Geometry: final body of the model. Coordinates: model frame, mm. Give positions to 0.01 mm unless a question says otherwise; leave off trailing zeros.
from build123d import *

# Parameters (mm, degrees)
BOSS_EXTRUDE1_DEPTH     = 3.175
SKETCH2_R               = 6.35
CUT_EXTRUDE1_DEPTH      = 4.1750001
CUT_EXTRUDE2_DEPTH      = 20.741500936
CUT_EXTRUDE2_DEPTH_BACK = 20.741500936


with BuildPart() as part:
    # Sketch1 → Boss-Extrude1 (new body)
    with BuildSketch(Plane.XY):
        with BuildLine():
            add(Edge.make_bspline(
                [(328.93, 0.4144518), (328.807900642, 0.516772717), (328.019000541, 0.420161926), (326.614170865, 0.815622818), (324.037900124, 1.060053788), (320.567272172, 1.584632638), (316.096583479, 2.170027594), (310.705215164, 2.891499965), (304.407193949, 3.70705594), (297.248126622, 4.61507178), (289.269853683, 5.599640546), (280.522284399, 6.647437516), (271.05918713, 7.745466949), (260.938835986, 8.878779448), (250.223661724, 10.033538187), (238.979802735, 11.195400912), (227.276553794, 12.349370833), (215.186101231, 13.479249677), (202.78290329, 14.570204468), (190.143565404, 15.603996393), (177.345750776, 16.563769435), (164.468478458, 17.43170464), (151.591090461, 18.189654233), (138.792862913, 18.818469572), (126.15283726, 19.301382712), (113.748578816, 19.622639213), (101.656743367, 19.766547691), (89.951630239, 19.721687508), (78.705404506, 19.479393557), (67.987291822, 19.033523951), (57.863264224, 18.382912366), (48.395544354, 17.529516447), (39.642067919, 16.480001255), (31.656190162, 15.24329661), (24.486303571, 13.832318834), (18.174431838, 12.263022231), (12.756441756, 10.550709399), (8.259860269, 8.711328155), (4.699027102, 6.757322776), (2.079421527, 4.684836659), (0.401585469, 2.443731656), (-0.187153107, 0), (0.401585469, -2.443731656), (2.079421527, -4.684836659), (4.699027102, -6.757322776), (8.259860269, -8.711328155), (12.756441756, -10.550709399), (18.174431838, -12.263022231), (24.486303571, -13.832318834), (31.656190162, -15.24329661), (39.642067919, -16.480001255), (48.395544354, -17.529516447), (57.863264224, -18.382912366), (67.987291822, -19.033523951), (78.705404506, -19.479393557), (89.951630239, -19.721687508), (101.656743367, -19.766547691), (113.748578816, -19.622639213), (126.15283726, -19.301382712), (138.792862913, -18.818469572), (151.591090461, -18.189654233), (164.468478458, -17.43170464), (177.345750776, -16.563769435), (190.143565404, -15.603996393), (202.78290329, -14.570204468), (215.186101231, -13.479249677), (227.276553794, -12.349370833), (238.979802735, -11.195400912), (250.223661724, -10.033538187), (260.938835986, -8.878779448), (271.05918713, -7.745466949), (280.522284399, -6.647437516), (289.269853683, -5.599640546), (297.248126622, -4.61507178), (304.407193949, -3.70705594), (310.705215164, -2.891499965), (316.096583479, -2.170027594), (320.567272172, -1.584632638), (324.037900124, -1.060053788), (326.614170865, -0.815622818), (328.019000541, -0.420161926), (329.127736254, -0.555940631), (329.127736254, 0.24874614), (328.93, 0.4144518)],
                knots=[0, 0, 0, 0, 0.000762215, 0.003044706, 0.006832246, 0.012101176, 0.018817536, 0.026939455, 0.036414848, 0.047184629, 0.059180413, 0.072327874, 0.086544061, 0.10174058, 0.117823336, 0.134691452, 0.152240154, 0.17036129, 0.188941008, 0.207865435, 0.227016078, 0.246275696, 0.265524943, 0.284644966, 0.303520118, 0.322034575, 0.340078353, 0.357542593, 0.374325482, 0.390329891, 0.40546389, 0.419643801, 0.432793371, 0.444843817, 0.455737921, 0.465428653, 0.47388632, 0.481101634, 0.487101684, 0.491975368, 0.495930678, 0.499382808, 0.502834938, 0.506790248, 0.511663932, 0.517663982, 0.524879296, 0.533336963, 0.543027695, 0.553921799, 0.565972245, 0.579121815, 0.593301726, 0.608435725, 0.624440134, 0.641223023, 0.658687263, 0.676731041, 0.695245498, 0.71412065, 0.733240673, 0.75248992, 0.771749538, 0.790900181, 0.809824608, 0.828404326, 0.846525462, 0.864074164, 0.88094228, 0.897025036, 0.912221555, 0.926437743, 0.939585203, 0.951580988, 0.962350768, 0.971826161, 0.979948081, 0.98666444, 0.991933371, 0.99572091, 0.998003402, 0.998765616, 1, 1, 1, 1], degree=3))
        make_face()
    extrude(amount=BOSS_EXTRUDE1_DEPTH)

    # Sketch2 → Cut-Extrude1 (cut, through all)
    with BuildSketch(Plane.XY.offset(3.175)):
        with Locations((88.9, 0)):
            Circle(SKETCH2_R)
        with Locations((165.1, 0)):
            Circle(SKETCH2_R)
    extrude(amount=-CUT_EXTRUDE1_DEPTH, mode=Mode.SUBTRACT)

    # Sketch3 → Cut-Extrude2 (cut, two sides)
    with BuildSketch(Plane(origin=(0, 0, 0), x_dir=(1, 0, 0), z_dir=(0, 1, 0))) as cut_extrude2_sk:
        Polygon((255.992242673, 0), (255.545593987, -3.175), (329.07830219, -3.175), (329.07830219, 0), align=None)
    extrude(amount=CUT_EXTRUDE2_DEPTH, mode=Mode.SUBTRACT)
    extrude(cut_extrude2_sk.sketch, amount=-CUT_EXTRUDE2_DEPTH_BACK, mode=Mode.SUBTRACT)

    # Sketch4 → Cut-Loft1 section 0
    with BuildSketch(Plane.XY.offset(3.175)):
        with BuildLine():
            Line((82.55, -19.515708197), (82.55, -16.251023077))
            Line((82.55, -16.251023077), (79.375, -16.251023077))
            add(Edge.make_bspline(
                [(79.375, 16.251023077), (72.770318552, 16.048049675), (66.176202719, 15.728304371), (56.30738853, 15.001567412), (53.021532705, 14.717888762), (46.459157571, 14.04734399), (43.182596705, 13.660937457), (38.276882967, 12.980450934), (36.643177419, 12.736779299), (33.379494145, 12.209172355), (31.748117674, 11.925180268), (28.498717967, 11.31067673), (26.880571377, 10.97988905), (23.660292552, 10.260780921), (22.058116365, 9.87261787), (18.875212279, 9.019251619), (17.293996052, 8.555526619), (14.162834442, 7.517257926), (12.611952901, 6.946125273), (10.325000489, 5.950076454), (9.567811499, 5.594025093), (8.461932827, 5.017489815), (8.097932617, 4.81777412), (7.381669561, 4.39922172), (7.029407018, 4.180395983), (6.339282138, 3.719594292), (6.001169966, 3.47795005), (5.346762375, 2.959692647), (5.02857237, 2.681117584), (4.439349211, 2.084395549), (4.164695388, 1.768387828), (3.820228536, 1.236176286), (3.718740433, 1.050561172), (3.59999989, 0.759299745), (3.565442077, 0.659141625), (3.509216677, 0.455376556), (3.487522742, 0.351764773), (3.459675736, 0.143592536), (3.453573255, 0.038940089), (3.461444597, -0.171798071), (3.474973766, -0.278422694), (3.536160139, -0.588423887), (3.603651886, -0.78636311), (3.780189655, -1.168677669), (3.889538593, -1.351988295), (4.129382817, -1.699026003), (4.261329389, -1.864987348), (4.67775825, -2.342961513), (4.979594961, -2.63427888), (5.614334641, -3.181856059), (5.947755344, -3.437548737), (6.980186178, -4.167859174), (7.695486627, -4.59881642), (9.156342741, -5.391257516), (9.902423269, -5.75319572), (11.414841066, -6.432708068), (12.181579116, -6.749404985), (13.73156777, -7.346635451), (14.514836956, -7.627179806), (16.093189665, -8.161972373), (16.88860874, -8.415184993), (18.482918694, -8.896317804), (19.282763312, -9.124717403), (21.688920309, -9.779957105), (23.302005405, -10.176164111), (26.541461257, -10.908476052), (28.167798474, -11.244732377), (33.062961618, -12.180447863), (36.350545365, -12.709560737), (42.938422768, -13.630876096), (46.23811967, -14.02274496), (52.84624923, -14.702163706), (56.154743063, -14.989298509), (66.090451195, -15.724271447), (72.727906329, -16.046777883), (79.375, -16.251023077)],
                knots=[0, 0, 0, 0, 0.125, 0.125, 0.1875, 0.1875, 0.25, 0.25, 0.28125, 0.28125, 0.3125, 0.3125, 0.34375, 0.34375, 0.375, 0.375, 0.40625, 0.40625, 0.4375, 0.4375, 0.453125, 0.453125, 0.4609375, 0.4609375, 0.46875, 0.46875, 0.4765625, 0.4765625, 0.484375, 0.484375, 0.4921875, 0.4921875, 0.49609375, 0.49609375, 0.498046875, 0.498046875, 0.5, 0.5, 0.501953125, 0.501953125, 0.50390625, 0.50390625, 0.5078125, 0.5078125, 0.51171875, 0.51171875, 0.515625, 0.515625, 0.5234375, 0.5234375, 0.53125, 0.53125, 0.546875, 0.546875, 0.5625, 0.5625, 0.578125, 0.578125, 0.59375, 0.59375, 0.609375, 0.609375, 0.625, 0.625, 0.65625, 0.65625, 0.6875, 0.6875, 0.75, 0.75, 0.8125, 0.8125, 0.875, 0.875, 1, 1, 1, 1], degree=3))
            Line((79.375, 16.251023077), (82.55, 16.251023077))
            Line((82.55, 16.251023077), (82.55, 19.515708197))
            Line((82.55, 19.515708197), (82.55, 26.856724286))
            Line((82.55, 26.856724286), (0.541465363, 30.021162049))
            Line((0.541465363, 30.021162049), (-2.146488993, -32.850745924))
            Line((-2.146488993, -32.850745924), (82.55, -25.525605715))
            Line((82.55, -25.525605715), (82.55, -19.515708197))
        make_face()
    # Sketch5 → Cut-Loft1 section 1
    with BuildSketch(Plane(origin=(0, 0, 0), x_dir=(-1, 0, 0), z_dir=(0, 0, -1))):
        with BuildLine():
            Line((-82.55, 16.286875084), (-82.55, 19.550482394))
            Line((-82.55, 19.550482394), (-82.55, 31.358919225))
            Line((-82.55, 31.358919225), (6.781155494, 29.861379368))
            Line((6.781155494, 29.861379368), (6.781155494, -36.639095207))
            Line((6.781155494, -36.639095207), (-82.55, -25.525605715))
            Line((-82.55, -25.525605715), (-82.55, -19.550482394))
            Line((-82.55, -19.550482394), (-82.55, -16.286875084))
            Line((-82.55, -16.286875084), (-79.375, -16.286825084))
            add(Edge.make_bspline(
                [(-79.375, -16.286825084), (-72.70273318, -16.083625481), (-66.040162391, -15.761734789), (-56.066904089, -15.02675589), (-52.74593973, -14.739468648), (-46.112636154, -14.059312037), (-42.800262288, -13.666866819), (-36.186801437, -12.743811384), (-32.886327655, -12.2135267), (-27.972128974, -11.275498707), (-26.339484745, -10.938349054), (-23.087489601, -10.204046758), (-21.46817298, -9.806739324), (-19.052762163, -9.149552861), (-18.249847199, -8.920461216), (-16.649429662, -8.437847637), (-15.850951917, -8.18383552), (-13.474510425, -7.379098548), (-11.914239449, -6.789912299), (-9.637231735, -5.767068515), (-8.888396164, -5.403819393), (-7.422171814, -4.608342986), (-6.704241471, -4.175660987), (-5.668127182, -3.442181611), (-5.333636046, -3.185395684), (-4.696951467, -2.635333166), (-4.394240594, -2.342641179), (-3.976788262, -1.862235899), (-3.844582818, -1.695403026), (-3.604511152, -1.346529706), (-3.495161032, -1.162204789), (-3.319211947, -0.777827241), (-3.252263911, -0.578820545), (-3.192281327, -0.267197855), (-3.179223041, -0.160018081), (-3.172509862, 0.051695952), (-3.179309615, 0.15678123), (-3.223308922, 0.470243795), (-3.283913969, 0.67718865), (-3.444877784, 1.066367796), (-3.547583565, 1.252275918), (-3.89542395, 1.785311832), (-4.171725698, 2.101726419), (-4.764220619, 2.699573748), (-5.08404298, 2.978749304), (-5.741470891, 3.497921226), (-6.081013127, 3.739966717), (-7.120428348, 4.432428384), (-7.84199373, 4.847705574), (-9.322334636, 5.617984146), (-10.082577048, 5.974865708), (-12.378451328, 6.97306267), (-13.935068025, 7.545295509), (-17.077417964, 8.585489689), (-18.664115765, 9.049996772), (-21.858212178, 9.904877668), (-23.466047551, 10.293687362), (-26.697720209, 11.014001073), (-28.321602434, 11.345344154), (-31.582558999, 11.960787009), (-33.219741649, 12.245183343), (-36.494895711, 12.773474887), (-38.134297303, 13.017428152), (-43.057081916, 13.69860264), (-46.345031773, 14.085282453), (-52.93019877, 14.756080578), (-56.227457948, 15.039733656), (-66.130500011, 15.766027755), (-72.74745852, 16.084987562), (-79.375, 16.286825084)],
                knots=[0, 0, 0, 0, 0.125, 0.125, 0.1875, 0.1875, 0.25, 0.25, 0.3125, 0.3125, 0.34375, 0.34375, 0.375, 0.375, 0.390625, 0.390625, 0.40625, 0.40625, 0.4375, 0.4375, 0.453125, 0.453125, 0.46875, 0.46875, 0.4765625, 0.4765625, 0.484375, 0.484375, 0.48828125, 0.48828125, 0.4921875, 0.4921875, 0.49609375, 0.49609375, 0.498046875, 0.498046875, 0.5, 0.5, 0.50390625, 0.50390625, 0.5078125, 0.5078125, 0.515625, 0.515625, 0.5234375, 0.5234375, 0.53125, 0.53125, 0.546875, 0.546875, 0.5625, 0.5625, 0.59375, 0.59375, 0.625, 0.625, 0.65625, 0.65625, 0.6875, 0.6875, 0.71875, 0.71875, 0.75, 0.75, 0.8125, 0.8125, 0.875, 0.875, 1, 1, 1, 1], degree=3))
            Line((-79.375, 16.286825084), (-82.55, 16.286875084))
        make_face()
    loft(mode=Mode.SUBTRACT)


solid = part.part
Item 1: Ray query, probe 1 along X at (y, z) = (-3, 2.25); probe 2 along X at (y, z) = (-3, 0.15); probe 3 along Y at (x, z) = (165.1, 1.55). Return the intervals inside material, ascending.
Values follow:
probe 1: x = 5.32 to 83.3, 94.5 to 159.5, 170.7 to 255.68
probe 2: x = 5.13 to 83.3, 94.5 to 159.5, 170.7 to 255.97
probe 3: y = -17.37 to -6.35, 6.35 to 17.37
Item 2: Section query A-A on y = 0. Give the number of separate pieces and of enclosed holes in the cut face, plus the area to 3 significant figures.
Values follow:
separate pieces: 3
enclosed holes: 0
area: 721 mm2
Item 3: Pin query (flat end, axial travel): pin 1 (1 mm diameter, centred on x = 50.5, z = 2, fed in from +Y); pin 2 (1.5 mm diameter, centred on x = 169, z = 0.5, fed in from -Y). Return the tip coordinate at first contact, or that it passes through.
Values follow:
pin 1: stops at y = 14.53
pin 2: stops at y = -17.17
Item 4: Draft query along Y for faces 1 (the face through (128, 0, 3.175)), 2 (the face through (171.157, 1.907, 1.61)). Return one class per face: +Y half, -Y half, draft (parallel to the pull), parting line (faces both ways), or undercut.
Values follow:
face 1: draft
face 2: undercut
